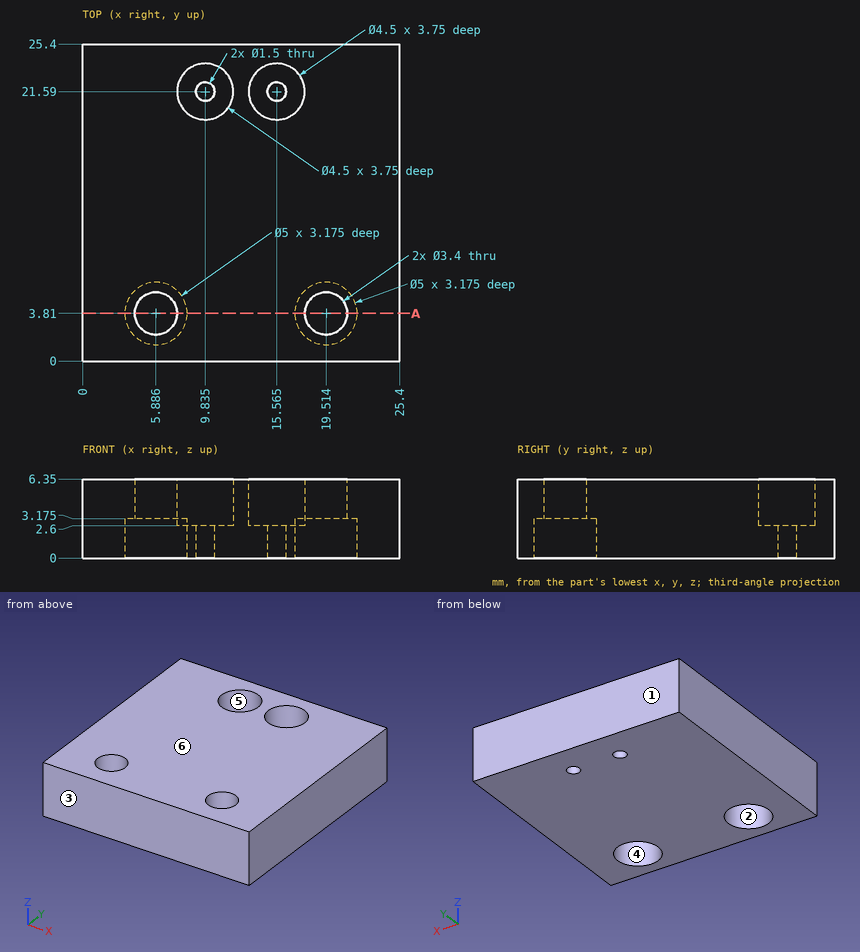
Design review of the part shown in the three views and the two pictorial views. Dimensions are in mm from the part's minimum x, y and z. A direction names the side the tool comes from. Give positions to 0.01 mm unless a question says otherwise; leave off trailing zeros. Return JSON: item names as keys, results as strings. Group by question number.
Item 1: Wall thickness on line 1 along X through (y, z) = (21.59, 1.7) (1 decimal); line 2 along X through (y, z) = (21.5, 3.75); line 3 along Y through (x, z) = (15.75, 4): over which ranges is each line inside the solid? List them lowest first.
Item 2: Clearance check with flat-ended pins moving along their axes: pin 1 Ø1.3 at (x, y) = (16.5, 21.5) entering from +Z; pin 2 Ø2.5 at (x, y) = (6.5, 3) entering from -Z (3 decimals). State where each tip first meets the part, or that it passes through.
Item 3: The part is to be moulded in two halves that separate along Y. For the marked faces 1, 2 and 3, say which applies: pulls with the +Y half, pulls with the -Y half, needs draft (parallel to the pull), parting line crosses it, or undercut.
Item 4: Tool access review of the marked faces 4, 5 and 6: name each direction out of +Z, -Z, +X, -X, +Y, -Y from which nothing blocks a thin tool from reaching the whole face with its end or side.
Item 5: Take a section at A-A (y = 3.81). Count the separate pieces of the cut face and the enclosed holes in it, plus the area to 3 significant figures.
Return value:
{
 "1": {"line 1": "x = 0 to 9.1, 10.6 to 14.8, 16.3 to 25.4", "line 2": "x = 0 to 7.59, 12.08 to 13.32, 17.81 to 25.4", "line 3": "y = 0 to 19.35, 23.83 to 25.4"},
 "2": {"pin 1": "stops at z = 2.6", "pin 2": "stops at z = 3.175"},
 "3": {"face 1": "pulls with the +Y half", "face 2": "undercut", "face 3": "pulls with the -Y half"},
 "4": {"face 4": "-Z", "face 5": "+Z", "face 6": "+Z, +X, -X, +Y, -Y"},
 "5": {"separate pieces": "3", "enclosed holes": "0", "area": "108 mm2"}
}
